Verification items for this drawing (mm, ordinates from the low corner). A direction names the side the tool comes from. Round coordinates to 2 decimals unless told otherwise and drop trailing zeros. Write each loop counter-clockwise with the first axis right and the second up, starting at its lowest first coordinate (ties: lowest second). Pieces come first, ordered by that corner, then holes. Notation, with made-up numbers: (6, 15.5) -> (22, 15.5) arc R27 cw to (22, 52.5) -> close; hole circle Ø3 at (47.5, -1). An arc over 180 degrees is marked (long way). One line per item, written item: value.
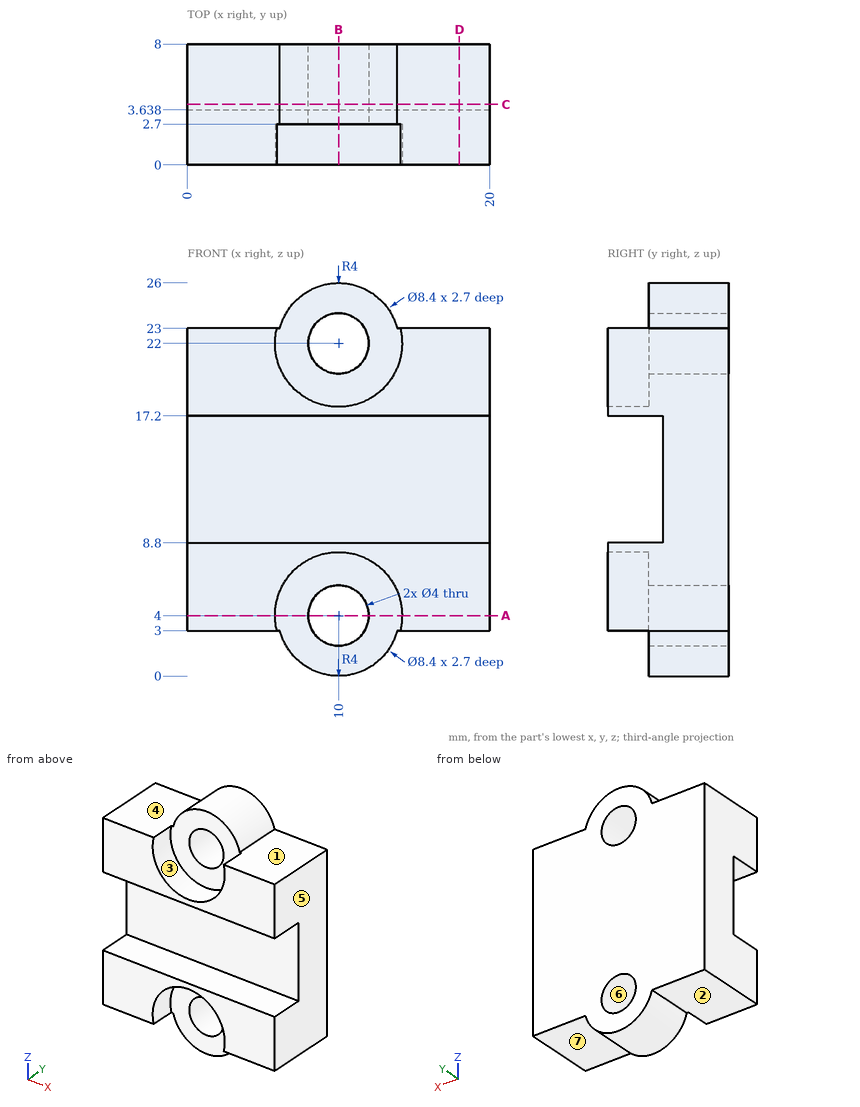
Item 1: Sectioned sample at A-A (z = 4). Enter the section's corners in (x, y), then the cut area to 3 significant figures.
Result set:
outline: (0, 0) -> (5.8, 0) -> (5.8, 2.7) -> (8, 2.7) -> (8, 8) -> (0, 8) -> close; (12, 2.7) -> (14.2, 2.7) -> (14.2, 0) -> (20, 0) -> (20, 8) -> (12, 8) -> close
area: 116 mm^2
Item 2: Depth check by flat-ended pin: pin 1 (3 mm diameter, centred on x = 8, y = 3.5, fed in from +Z); pin 2 (4.5 mm diameter, centred on x = 10, z = 4, fed in from -Y); pin 3 (3 mm diameter, centred on x = 9.5, y = 2, fed in from -Z); pin 4 (1.8 mm diameter, centred on x = 7, y = 2, fed in from +Z) (1 decimal). Enter the tip coordinate at first touch or a pass-through.
Result set:
pin 1: z = 25.97
pin 2: y = 2.7
pin 3: z = 0
pin 4: z = 25.2
Item 3: Material ranges on line 1 along X through (y, z) = (2.05, 4); line 2 along Z through (x, y) = (17.5, 1.25); line 3 along Z through (x, y) = (10, 1.1), recorded low to high.
Result set:
line 1: 0 to 5.8, 14.2 to 20
line 2: 3 to 8.8, 17.2 to 23
line 3: 8.2 to 8.8, 17.2 to 17.8
Item 4: Tool access check on the marked faces 1, 2, 3 and 4. Record the directions out of +Z, -Z, +X, -X, +Y, -Y that give a thin tool (end or side, any length) a straight path to the whole face; none if there is none.
Result set:
face 1: +Z, +X, +Y, -Y
face 2: -Z, -X, +Y, -Y
face 3: -Y
face 4: +Z, -X, +Y, -Y
Item 5: Sectioned sample at C-C (y = 4). Enter the section's corners in (x, z).
Result set:
outline: (0, 3) -> (6.13, 3) arc R4 ccw to (13.87, 3) -> (20, 3) -> (20, 23) -> (13.87, 23) arc R4 ccw to (6.13, 23) -> (0, 23) -> close; hole circle Ø4 at (10, 4); hole circle Ø4 at (10, 22)
Item 6: Release check for a two-part mould opening along Z. For the marked faces 5, 6 and 7 record: pulls with the +Z half, pulls with the -Z half, needs draft (parallel to the pull), parting line crosses it, or undercut.
Result set:
face 5: needs draft
face 6: undercut
face 7: pulls with the -Z half
Item 7: Sectioned sample at D-D (x = 18). Enter the section's corners in (y, z).
Result set:
outline: (0, 3) -> (8, 3) -> (8, 23) -> (0, 23) -> (0, 17.2) -> (3.64, 17.2) -> (3.64, 8.8) -> (0, 8.8) -> close
Item 8: Sectioned sample at B-B (x = 10). Enter the section's corners in (y, z).
Result set:
outline: (0, 8.2) -> (2.7, 8.2) -> (2.7, 6) -> (8, 6) -> (8, 20) -> (2.7, 20) -> (2.7, 17.8) -> (0, 17.8) -> (0, 17.2) -> (3.64, 17.2) -> (3.64, 8.8) -> (0, 8.8) -> close; (2.7, 0) -> (8, 0) -> (8, 2) -> (2.7, 2) -> close; (2.7, 24) -> (8, 24) -> (8, 26) -> (2.7, 26) -> close
